Autodesk Fusion 360 part; units mm, degrees
sketch "草图1" plane through (0, 0, 0) normal (0, 0, 1) x (1, 0, 0)
  line L0 (7.5, 60) -> (7.5, 75)
  circle A0 centre (-42.5, 42.5) radius 32.5 construction
  arc A1 (-7.5, 60) -> (7.5, 60) centre (0, 60) ccw
  circle A2 centre (42.5, 42.5) radius 32.5 construction
  circle A3 centre (-10, 80) radius 1.05
  line L1 (-7.5, 75) -> (-7.5, 60)
  line L2 (57.8614, 83) -> (0, 83)
  line L3 (0, 60) -> (0, 75) construction
  circle A4 centre (10, 80) radius 1.05
  circle A5 centre (42.5, -42.5) radius 32.5 construction
  circle A6 centre (-42.5, -42.5) radius 32.5 construction
  arc A7 (7.5, 75) -> (-7.5, 75) centre (0, 75) ccw construction
  line L4 (7.5, 75) -> (7.5, 78)
  line L5 (7.5, 78) -> (57.2046, 78)
  line L6 (0, 0) -> (89.0494, 89.0494) construction
  line L7 (57.2046, 78) -> (67.6023, 67.6023)
  line L8 (57.8614, 83) -> (70.4307, 70.4307)
  line L9 (-57.8614, 83) -> (0, 83)
  line L10 (-57.8614, 83) -> (-70.4307, 70.4307)
  line L11 (-57.2046, 78) -> (-67.6023, 67.6023)
  line L12 (-7.5, 78) -> (-57.2046, 78)
  line L13 (-7.5, 75) -> (-7.5, 78)
  line L14 (-4, 75) -> (-4, 60)
  arc A8 (-4, 60) -> (4, 60) centre (0, 60) ccw
  line L15 (4, 60) -> (4, 75)
  arc A9 (4, 75) -> (-4, 75) centre (0, 75) ccw
  line L16 (0, 75) -> (0, 60) construction
  line L17 (-83, -57.8614) -> (-70.4307, -70.4307)
  line L18 (-83, -57.8614) -> (-83, 0)
  line L19 (-83, 57.8614) -> (-83, 0)
  line L20 (-83, 57.8614) -> (-70.4307, 70.4307)
  line L21 (-78, 57.2046) -> (-67.6023, 67.6023)
  line L22 (-78, 7.5) -> (-78, 57.2046)
  line L23 (-75, 7.5) -> (-78, 7.5)
  line L24 (-60, 7.5) -> (-75, 7.5)
  arc A10 (-60, -7.5) -> (-60, 7.5) centre (-60, 0) ccw
  line L25 (-75, -7.5) -> (-60, -7.5)
  line L26 (-75, -7.5) -> (-78, -7.5)
  line L27 (-78, -7.5) -> (-78, -57.2046)
  line L28 (-78, -57.2046) -> (-67.6023, -67.6023)
  line L29 (-75, -4) -> (-60, -4)
  arc A11 (-75, 4) -> (-75, -4) centre (-75, 0) ccw
  line L30 (-60, 4) -> (-75, 4)
  arc A12 (-60, -4) -> (-60, 4) centre (-60, 0) ccw
  circle A13 centre (-80, -10) radius 1.05
  circle A14 centre (-80, 10) radius 1.05
  line L31 (57.8614, -83) -> (70.4307, -70.4307)
  line L32 (57.8614, -83) -> (0, -83)
  line L33 (-57.8614, -83) -> (0, -83)
  line L34 (-57.8614, -83) -> (-70.4307, -70.4307)
  line L35 (-57.2046, -78) -> (-67.6023, -67.6023)
  line L36 (-7.5, -78) -> (-57.2046, -78)
  line L37 (-7.5, -75) -> (-7.5, -78)
  line L38 (-7.5, -60) -> (-7.5, -75)
  arc A15 (7.5, -60) -> (-7.5, -60) centre (0, -60) ccw
  line L39 (7.5, -75) -> (7.5, -60)
  line L40 (7.5, -75) -> (7.5, -78)
  line L41 (7.5, -78) -> (57.2046, -78)
  line L42 (57.2046, -78) -> (67.6023, -67.6023)
  line L43 (4, -75) -> (4, -60)
  arc A16 (-4, -75) -> (4, -75) centre (0, -75) ccw
  line L44 (-4, -60) -> (-4, -75)
  arc A17 (4, -60) -> (-4, -60) centre (0, -60) ccw
  circle A18 centre (10, -80) radius 1.05
  circle A19 centre (-10, -80) radius 1.05
  line L45 (83, 57.8614) -> (70.4307, 70.4307)
  line L46 (83, 57.8614) -> (83, 0)
  line L47 (83, -57.8614) -> (83, 0)
  line L48 (83, -57.8614) -> (70.4307, -70.4307)
  line L49 (78, -57.2046) -> (67.6023, -67.6023)
  line L50 (78, -7.5) -> (78, -57.2046)
  line L51 (75, -7.5) -> (78, -7.5)
  line L52 (60, -7.5) -> (75, -7.5)
  arc A20 (60, 7.5) -> (60, -7.5) centre (60, 0) ccw
  line L53 (75, 7.5) -> (60, 7.5)
  line L54 (75, 7.5) -> (78, 7.5)
  line L55 (78, 7.5) -> (78, 57.2046)
  line L56 (78, 57.2046) -> (67.6023, 67.6023)
  line L57 (75, 4) -> (60, 4)
  arc A21 (75, -4) -> (75, 4) centre (75, 0) ccw
  line L58 (60, -4) -> (75, -4)
  arc A22 (60, 4) -> (60, -4) centre (60, 0) ccw
  circle A23 centre (80, 10) radius 1.05
  circle A24 centre (80, -10) radius 1.05
  dimension "d3" = 65
  dimension "d4" = 65
  dimension "d5" = 65
  dimension "d6" = 65
  dimension "d7" = 15
  dimension "d8" = 15
  dimension "d10" = 2.1
  dimension "d11" = 5
  dimension "d12" = 10
  dimension "d15" = 3
  dimension "d16" = 2
  dimension "d17" = 60
  dimension "d18" = 35.5
  dimension "d19" = 4
  dimension "d20" = 8
  dimension "d22" = 360
extrude "拉伸1" add sketch "草图1" along normal blind 2
fillet "圆角1" radius 2 16 edges at (-57.2046, 78, 1) (57.2046, 78, 1) (78, 57.2046, 1) (-7.5, 78, 1) (7.5, 78, 1) (78, 7.5, 1) (78, -7.5, 1) (78, -57.2046, 1) (57.2046, -78, 1) (7.5, -78, 1) (-7.5, -78, 1) (-57.2046, -78, 1) (-78, -57.2046, 1) (-78, -7.5, 1) (-78, 7.5, 1) (-78, 57.2046, 1)
fillet "圆角2" radius 2 8 edges at (83, -57.8614, 1) (57.8614, -83, 1) (-57.8614, -83, 1) (-83, -57.8614, 1) (-83, 57.8614, 1) (-57.8614, 83, 1) (57.8614, 83, 1) (83, 57.8614, 1)
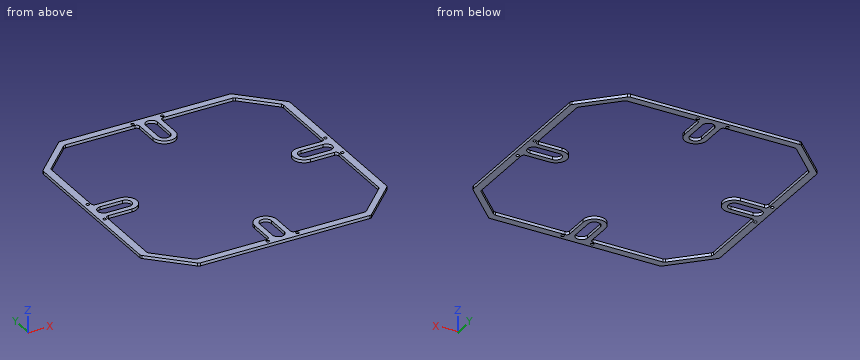
Build history of the part. All positions in model axes, mm. Coordinates: 2 decimals unless noted, no trailing zeros. Order: outer loops, then holes, each group sorted by start corner. A loop starts at its lowest first (then second) coordinate and runs counter-clockwise, first axis right, second up. Notation, with made-up numbers: M 29.5,-29.5 L 45.5,-29.5 A16 cw 45.5,-16.5 Z; hole C 56.5,56.5 d3. An arc over 180 degrees is marked long. One line per question, with ' | ' between items. Start each with the question number.
1. Cut at A-A (y = 0). Write the cut outline in (x, z), plus the area to 3 significant figures.
2. Cut at C-C (x = 67). Write the cut outline in (y, z), plus the area to 3 significant figures.
3. Flat gauge pins, fed straight in: P1, Ø1, axis at y = -69.5, z = 1, coming from the -X side; P2, Ø0.6, axis at x = -64, z = 1.5, coming from the +Y side; P3, Ø0.6, axis at y = 64.5, z = 1, coming from the +X side. Where does each tip first touch, or does it go through?
4. Wall check: line 1 along Y through (x, z) = (10, 1.2); line 2 along Y through (x, z) = (0, 1.55); line 3 along Y through (x, z) = (34, 0.2). Give the ranges that are in metal, low to high. Write a range as [from, to].
5. Cut at B-B (y = 44.5). Write the cut outline in (x, z).
The answers:
1) outline: M -83,0 L -79,0 L -79,2 L -83,2 Z; M -56,0 L -52.5,0 L -52.5,2 L -56,2 Z; M 52.5,0 L 56,0 L 56,2 L 52.5,2 Z; M 79,0 L 83,0 L 83,2 L 79,2 Z | area: 30.0 mm2
2) outline: M -73.86,0 L -68.2,0 L -68.2,2 L -73.86,2 Z; M -7.5,0 L -4,0 L -4,2 L -7.5,2 Z; M 4,0 L 7.5,0 L 7.5,2 L 4,2 Z; M 68.2,0 L 73.86,0 L 73.86,2 L 68.2,2 Z | area: 36.6 mm2
3) P1: stops at x = -71.86 | P2: stops at y = 77.16 | P3: stops at x = 76.66
4) line 1: y = [-83, -81.05], [-78.95, -78], [78, 78.95], [81.05, 83] | line 2: y = [-83, -79], [-56, -52.5], [52.5, 56], [79, 83] | line 3: y = [-83, -78], [78, 83]
5) outline: M -83,0 L -78,0 L -78,2 L -83,2 Z; M 78,0 L 83,0 L 83,2 L 78,2 Z
